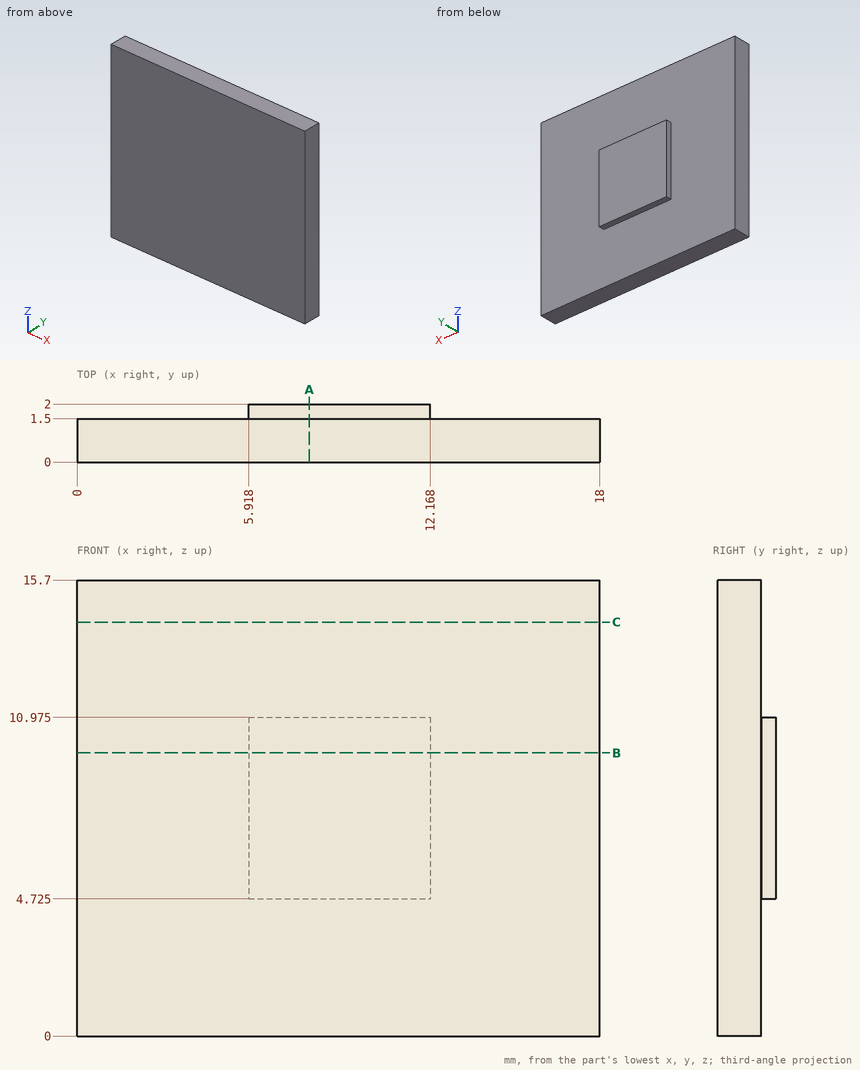
For this review, use the dimensioned drawing (mm, ordinates from the lowest corner) and the shaded views. Give positions to 0.01 mm unless a question says otherwise; leave off trailing zeros. Order: outer loops, then holes, each group sorted by start corner. A loop starts at its lowest first (then second) coordinate and runs counter-clockwise, first axis right, second up. Notation, with made-up numbers: M -34,-2 L -30,-2 A29 ccw -30,23 Z; hole C 16,10 d5. An arc over 180 degrees is marked long. One line per question, with ' | ' between items. Start each with the question number.
1) Clearance check with flat-ended pins moving along their axes: P1, Ø0.6, axis at x = 9, y = 2, coming from the +Z side (3 decimals); P2, Ø4, axis at x = 2, z = 3, coming from the +Y side. State where each tip first meets the part, or that it passes through.
2) Consider section C-C, the plane z = 14.25. Give the boundary of the cut face in (x, y).
3) Consider section B-B, the plane z = 9.75. Give the boundary of the cut face in (x, y), then the cut area to 3 significant figures.
4) Wall thickness on L1, parallel to Y at x = 5, z = 2.25; L2, parallel to X at y = 1.9, z = 7.5: over which ranges is each line inside the solid? List them lowest first. Write a range as from..to.
5) Consider section A-A, the plane x = 8. Give the boundary of the cut face in (y, z) (1 decimal), then the cut area to 3 significant figures.
Found:
1) P1: stops at z = 10.975 | P2: stops at y = 1.5
2) outline: M 0,0 L 18,0 L 18,1.5 L 0,1.5 Z
3) outline: M 0,0 L 18,0 L 18,1.5 L 12.17,1.5 L 12.17,2 L 5.92,2 L 5.92,1.5 L 0,1.5 Z | area: 30.1 mm²
4) L1: y = 0..1.5 | L2: x = 5.92..12.17
5) outline: M 0,0 L 1.5,0 L 1.5,4.7 L 2,4.7 L 2,11 L 1.5,11 L 1.5,15.7 L 0,15.7 Z | area: 26.7 mm²
